The figure shows three views and two pictorial views of one solid part (mm, origin at its lowest corner). Answer the questions. A direction names the side the tool comes from. Round coordinates to 2 decimals unless told otherwise and drop trailing zeros. Order: outer loops, then holes, each group sorted by start corner. A loop starts at its lowest first (then second) coordinate and runs counter-clockwise, first axis right, second up. Notation, with made-up numbers: (15, 18.25) -> (20, 18.25) arc R21 ccw to (20, 51.25) -> close; hole circle Ø6 at (23, -22.75). An arc over 180 degrees is marked (long way). Answer as a JSON object with one key per item and string values. Group by question number.
Item 1: Section B-B, the plane z = 16.5 is taken. Write down the section's boundary in (x, y) (1 decimal), plus the area to 3 significant figures.
Item 2: The mould has two halves that part along Z. Classify the marked faces 3, 4 and 5: pulls with the +Z half, pulls with the -Z half, needs draft (parallel to the pull), parting line crosses it, or undercut.
Item 3: Consider probe 1 along Z at (x, y) = (17, 6.5); probe 2 along X at (y, z) = (2, 11) (1 decimal); probe 3 along Z at (x, y) = (18, 1.5) (1 decimal). Determine where each line is inside the solid, lowest interval first. Write a range as from..to.
Item 4: Given P1, Ø1.5, axis at x = 9.5, y = 5.5, coming from the -Z side; P2, Ø4, axis at y = 6.5, z = 8.5, coming from the +X side, each flat-ended and moving along its own axis, determine where each tip first touches the part or whether it passes through.
Item 5: Section A-A, the plane y = 1 is taken. Write down the section's boundary in (x, z).
Item 6: For the marked faces 1 and 2, determine the directions among +Z, -Z, +X, -X, +Y, -Y from which every point of the face is accessible in a straight line to the end or side of a thin tool.
Item 7: Section C-C, the plane x = 14.5 is taken. Write down the section's boundary in (y, z).
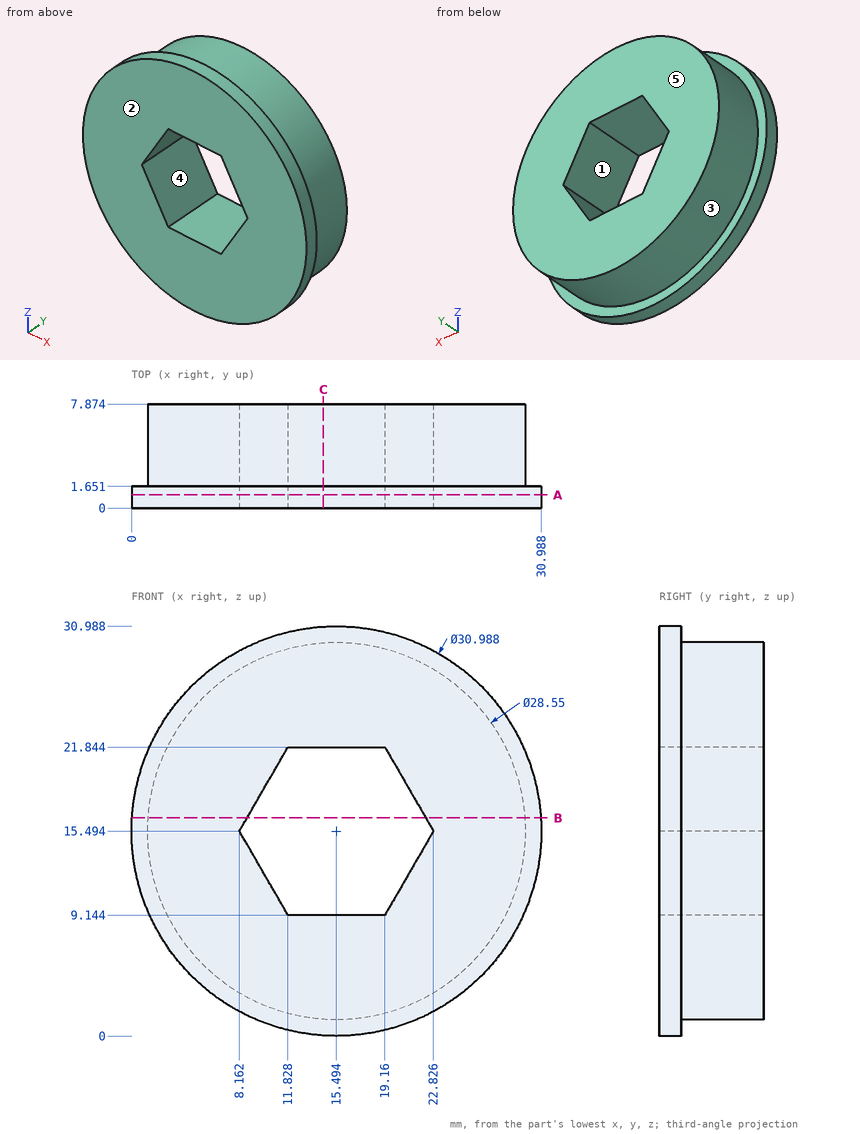
Values found:
{
 "1": {"outline": "(0, 0) -> (8.7, 0) -> (8.7, 7.9) -> (1.3, 7.9) -> (1.3, 1.7) -> (0, 1.7) -> close; (22.2, 0) -> (31, 0) -> (31, 1.7) -> (29.7, 1.7) -> (29.7, 7.9) -> (22.2, 7.9) -> close", "area": "122 mm2"},
 "2": {"face 3": "parting line crosses it", "face 4": "undercut", "face 5": "needs draft"},
 "3": {"probe 1": "1.3..9.14, 21.84..29.69", "probe 2": "1.9..10.8, 20.2..29", "probe 3": "0.2..9.1, 21.8..30.8"},
 "4": {"P1": "z = 2.22", "P2": "x = 28.87"},
 "5": {"outline": "circle Ø30.99 at (15.49, 15.49); hole (8.16, 15.49) -> (11.83, 9.14) -> (19.16, 9.14) -> (22.83, 15.49) -> (19.16, 21.84) -> (11.83, 21.84) -> close"},
 "6": {"face 1": "+Y, -Y", "face 2": "+Z, -Z, +X, -X, -Y"},
 "7": {"outline": "(0, 0.03) -> (1.65, 0.03) -> (1.65, 1.25) -> (7.87, 1.25) -> (7.87, 9.14) -> (0, 9.14) -> close; (0, 21.84) -> (7.87, 21.84) -> (7.87, 29.73) -> (1.65, 29.73) -> (1.65, 30.96) -> (0, 30.96) -> close"}
}
